Model file for the job. Use its own axes, mm. A direction names the side the tool comes from. Round coordinates to 2 decimals unless told otherwise and drop trailing zeros. Order: outer loops, then holes, each group sorted by start corner. A loop starts at its lowest first (then second) coordinate and runs counter-clockwise, first axis right, second up. Notation, with made-up numbers: (33, -23.5) -> (82, -23.5) arc R30 ccw to (82, 10.5) -> close; hole circle Ø10 at (31.5, 59.5). An arc over 180 degrees is marked (long way). Use CSV: the item, a comma, the result in double quotes.
```python
from build123d import *

# Parameters (mm, degrees)
BOSS_EXTRUDE1_DEPTH = 3.5
SKETCH2_R           = 1.5
CUT_EXTRUDE1_DEPTH  = 3.5
SKETCH3_W           = 23
SKETCH3_H           = 10.283770076
CUT_EXTRUDE2_DEPTH  = 2
CUT_EXTRUDE6_DEPTH  = 3.5


with BuildPart() as part:
    # Sketch1 → Boss-Extrude1 (new body)
    with BuildSketch(Plane(origin=(0, 0, 0), x_dir=(1, 0, 0), z_dir=(0, 1, 0))):
        with BuildLine():
            Line((-20.62248996, 7.565261044), (54.37751004, 7.565261044))
            ThreePointArc((54.37751004, 7.565261044), (57.913043946, 6.10079495), (59.37751004, 2.565261044))
            Line((59.37751004, 2.565261044), (59.37751004, -42.434738956))
            ThreePointArc((59.37751004, -42.434738956), (57.913043946, -45.970272862), (54.37751004, -47.434738956))
            Line((54.37751004, -47.434738956), (-20.62248996, -47.434738956))
            ThreePointArc((-20.62248996, -47.434738956), (-24.158023866, -45.970272862), (-25.62248996, -42.434738956))
            Line((-25.62248996, -42.434738956), (-25.62248996, 2.565261044))
            ThreePointArc((-25.62248996, 2.565261044), (-24.158023866, 6.10079495), (-20.62248996, 7.565261044))
        make_face()
    extrude(amount=BOSS_EXTRUDE1_DEPTH)

    # Sketch2 → Cut-Extrude1 (cut)
    with BuildSketch(Plane(origin=(0, 3.5, 0), x_dir=(1, 0, 0), z_dir=(0, 1, 0))):
        with Locations((-22.187566987, 3.802718615)):
            Circle(SKETCH2_R)
        with Locations((55.412433013, 3.947865339)):
            Circle(SKETCH2_R)
        with Locations((55.766505812, -43.552134661)):
            Circle(SKETCH2_R)
        with Locations((-21.775437199, -43.697281385)):
            Circle(SKETCH2_R)
    extrude(amount=-CUT_EXTRUDE1_DEPTH, mode=Mode.SUBTRACT)

    # Sketch3 → Cut-Extrude2 (cut)
    with BuildSketch(Plane(origin=(0, 3.5, 0), x_dir=(1, 0, 0), z_dir=(0, 1, 0))):
        with Locations((16.87751004, -42.292853918)):
            Rectangle(SKETCH3_W, SKETCH3_H)
        Polygon((59.37751004, -2.947281385), (-25.62248996, -2.947281385), (-25.62248996, -37.15096888), (5.37751004, -37.15096888), (28.37751004, -37.15096888), (59.37751004, -37.15096888), align=None)
    extrude(amount=-CUT_EXTRUDE2_DEPTH, mode=Mode.SUBTRACT)

    # Sketch9 → Cut-Extrude6 (cut)
    with BuildSketch(Plane(origin=(0, 3.5, 0), x_dir=(1, 0, 0), z_dir=(0, 1, 0))):
        with BuildLine():
            Line((38.139406345, 7.565261044), (51.719818859, 7.565261044))
            Line((51.719818859, 7.565261044), (51.90057812, 7.565261044))
            ThreePointArc((51.90057812, 7.565261044), (45.019992232, 0.684675157), (38.139406345, 7.565261044))
        make_face()
    extrude(amount=-CUT_EXTRUDE6_DEPTH, mode=Mode.SUBTRACT)


solid = part.part
```
Q1. Cut at C-C (x = 26.5). Give the cut face in (y, z), plus the area to 3 significant figures.
From the geometry:
outline,"(0, -7.57) -> (3.5, -7.57) -> (3.5, 2.95) -> (1.5, 2.95) -> (1.5, 47.43) -> (0, 47.43) -> close"
area,"104 mm²"
Q2. Cut at B-B (y = 2.4). Give the cut face in (x, z).
From the geometry:
outline,"(-25.62, -2.57) arc R5 ccw to (-20.62, -7.57) -> (38.14, -7.57) arc R6.88 cw to (51.9, -7.57) -> (54.38, -7.57) arc R5 ccw to (59.38, -2.57) -> (59.38, 2.95) -> (-25.62, 2.95) -> close; (-25.62, 37.15) -> (5.38, 37.15) -> (5.38, 47.43) -> (-20.62, 47.43) arc R5 ccw to (-25.62, 42.43) -> close; (28.38, 37.15) -> (59.38, 37.15) -> (59.38, 42.43) arc R5 ccw to (54.38, 47.43) -> (28.38, 47.43) -> close; hole circle Ø3 at (-22.19, -3.8); hole circle Ø3 at (-21.78, 43.7); hole circle Ø3 at (55.41, -3.95); hole circle Ø3 at (55.77, 43.55)"
Q3. Cut at D-D (z = 33). Give the cut face in (x, y).
From the geometry:
outline,"(-25.62, 0) -> (59.38, 0) -> (59.38, 1.5) -> (-25.62, 1.5) -> close"
Q4. Mould opens along X. For faces 1 (the flat face through (17, 1, 47.435)), 2 (the cylindrical face through (45.171, 1.774, -0.686)), 3 (the cylindrical face through (-24.12, 1.73, 46.01)) say: +X half, -X half, draft (parallel to the pull), parting line (faces both ways), or undercut.
From the geometry:
face 1,"draft"
face 2,"undercut"
face 3,"-X half"
Q5. Probe line 1 along X through (y, z) = (2.9, 40); line 2 along X through (y, z) = (2.2, 44.5); line 3 along Z through (x, y) = (37, 3.35). List the from-to ranges inside material, lowest first.
From the geometry:
line 1,"x = -25.62 to 5.38, 28.38 to 59.38"
line 2,"x = -25.18 to -23.04, -20.51 to 5.38, 28.38 to 54.6, 56.93 to 58.93"
line 3,"z = -7.57 to 2.95, 37.15 to 47.43"
Q6. Which spindle directions (+Z, -Z, +X, -X, +Y, -Y) get a long thin tool onto all of the face, cutting with end or side? Do faces 4 (the flat face through (44, 3, 37.151)), 5 (the flat face through (5.378, 3, 42)), 6 (the cylindrical face through (56.105, 1.774, -2.617)). Say none if no direction does.
From the geometry:
face 4,"+X, -X, +Y"
face 5,"+Z, +Y"
face 6,"+Y, -Y"
Q7. Cut at A-A (x = -18). Give the cut face in (y, z).
From the geometry:
outline,"(0, -7.57) -> (3.5, -7.57) -> (3.5, 2.95) -> (1.5, 2.95) -> (1.5, 37.15) -> (3.5, 37.15) -> (3.5, 47.43) -> (0, 47.43) -> close"
Q8. Pin check, flat tips, straight feed: pin 1 (13.5 mm diameter, centred on x = 5.5, z = 21, fed in from +Y); pin 2 (1.6 mm diameter, centred on y = 2, z = 44, fed in from -X); pin 3 (2 mm diameter, centred on x = 43.5, y = 2, fed in from -Z). Stop position of each tip, or through.
From the geometry:
pin 1,"stops at y = 1.5"
pin 2,"stops at x = -25.56"
pin 3,"stops at z = -1.16"
